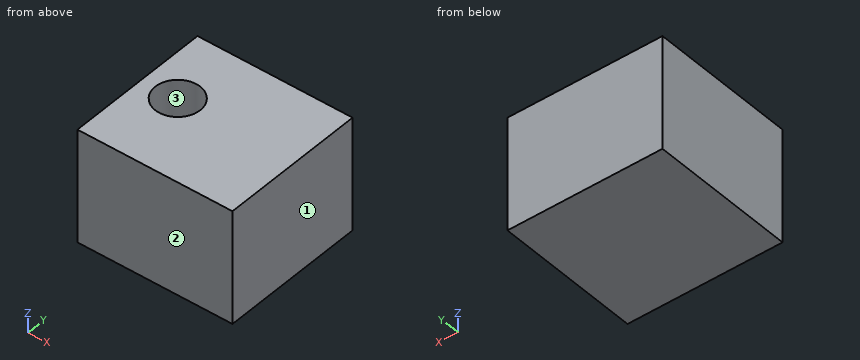
from build123d import *

# Parameters (mm, degrees)
F0_W     = 99.467852
F0_H     = 72.783896
F1_DEPTH = 93.726
F2_R     = 14.41662
F3_DEPTH = 25.4


with BuildPart() as f1:
    # F0 (on Front) → F1 (new body)
    with BuildSketch(Plane.XZ):
        with Locations((-12.687225, 5.47232)):
            Rectangle(F0_W, F0_H)
    extrude(amount=F1_DEPTH)

    # F2 (on face) → F3 (cut)
    with BuildSketch(Plane.XY.offset(41.864268)):
        with Locations((-39.331704, -43.508075)):
            Circle(F2_R)
    extrude(amount=-F3_DEPTH, mode=Mode.SUBTRACT)


with BuildPart() as f1_1:
    # F4: moved
    add(f1.part.moved(Location((13.716, -14.986, 4.064))))


solid = f1_1.part
Could you check a few things on this model? Use its own coordinates, in mm. Face numbers are marked on the shaded views. Coordinates: 2 decimals unless noted, no trailing zeros. Order: outer loops, then holes, each group sorted by start corner. A loop starts at its lowest first (then second) coordinate and runs counter-clockwise, first axis right, second up. Notation, with made-up numbers: (21, 37.5) - (61, 37.5) arc R21 cw to (61, 56.5) - close; hole circle Ø9 at (62, -39). An arc over 180 degrees is marked (long way). Answer in a Markdown table with one row per item. Add a question column.
(1) If we section it at C-C, the plane z = 40: Please give me the cut outline in (x, y), then the cut area to 3 significant figures.
(2) If we section it at B-B, the plane x = -33.5: Please give me the cut outline in (y, z), then the cut area to 3 significant figures.
(3) I need wall thicknesses on L1, parallel to Y at x = -38, z = 21.5; L2, parallel to Z at x = -29, y = -65.5; L3, parallel to Y at x = -14.5, z = 27.5. Which ranges of each line are inside material? Lowest first, please.
(4) Will this pin go through, and if not, where does the flat tip stop? pin 1 (8.5 mm diameter, centred on x = -23.5, y = -52.5, fed in from +Z).
(5) If we mould it in two halves opening along X, with no side actions, what happens to the marked faces 1, 2 and 3? For each: released by +X, released by -X, zero draft, split by the parting line, or undercut.
(6) If we section it at A-A, the plane y = -50: Please give me the cut outline in (x, z).
Results are:
| question | item | result |
|---|---|---|
| 1 | outline | (-48.71, -108.71) - (50.76, -108.71) - (50.76, -14.99) - (-48.71, -14.99) - close; hole circle Ø28.83 at (-25.62, -58.49) |
| 1 | area | 8,670 mm2 |
| 2 | outline | (-108.71, -26.86) - (-14.99, -26.86) - (-14.99, 45.93) - (-46.42, 45.93) - (-46.42, 20.53) - (-70.56, 20.53) - (-70.56, 45.93) - (-108.71, 45.93) - close |
| 2 | area | 6,210 mm2 |
| 3 | L1 | y = -108.71 to -65.87, -51.11 to -14.99 |
| 3 | L2 | z = -26.86 to 20.53 |
| 3 | L3 | y = -108.71 to -67.67, -49.31 to -14.99 |
| 4 | pin 1 | stops at z = 20.53 |
| 5 | face 1 | released by +X |
| 5 | face 2 | zero draft |
| 5 | face 3 | undercut |
| 6 | outline | (-48.71, -26.86) - (50.76, -26.86) - (50.76, 45.93) - (-13.97, 45.93) - (-13.97, 20.53) - (-37.26, 20.53) - (-37.26, 45.93) - (-48.71, 45.93) - close |
